Geometry check sheet. Reference: the model listing, model coordinates, mm. A direction names the side the tool comes from. Coordinates: 2 decimals unless noted, no trailing zeros. Write each loop counter-clockwise with the first axis right and the second up, starting at its lowest first coordinate (ties: lowest second). Pieces come first, ordered by that corner, then holes. Notation, with made-up numbers: M 50,5 L 104,5 A25 ccw 104,39 Z; hole C 45,5 d1. An arc over 180 degrees is marked long. Write each question's results on one line, items separated by ' | '.
Autodesk Inventor part; units mm, degrees
ref_plane "YZ Plane" through (0, 0, 0) normal (1, 0, 0) x (0, 1, 0)
ref_plane "XZ Plane" through (0, 0, 0) normal (0, 1, 0) x (-1, 0, 0)
ref_plane "XY Plane" through (0, 0, 0) normal (0, 0, 1) x (1, 0, 0)
sketch "Sketch1" plane through (0, 0, 0) normal (0, 1, 0) x (-1, 0, 0)
  line L0 (0, 0) -> (180, 0)
  line L1 (180, 0) -> (180, -60)
  line L2 (180, -60) -> (0, -60)
  line L3 (0, -60) -> (0, 0)
  dimension "d0" = 180
  dimension "d34" = 60
extrude "Plate1" add sketch "Sketch1" along normal blind 3
sketch "Sketch2" plane through (0, 3, 0) normal (0, 1, 0) x (1, 0, 0)
  line L0 (0, 60) -> (0, 0)
  line L1 (-180, 0) -> (-180, 60)
  line L2 (-133, 18.2) -> (-47, 18.2) construction
  line L3 (-180, 60) -> (0, 60) construction
  circle A0 centre (-103, 147.6372) radius 2
  circle A1 centre (-47, 147.6372) radius 2
  line L4 (-40, 142.6372) -> (-110, 142.6372)
  line L5 (-110, 142.6372) -> (-110, 152.6372)
  line L6 (-110, 152.6372) -> (-40, 152.6372)
  line L7 (-40, 152.6372) -> (-40, 142.6372)
  circle A2 centre (-103, 162.6372) radius 2
  circle A3 centre (-47, 162.6372) radius 2
  line L8 (-40, 157.6372) -> (-110, 157.6372)
  line L9 (-110, 157.6372) -> (-110, 167.6372)
  line L10 (-110, 167.6372) -> (-40, 167.6372)
  line L11 (-40, 167.6372) -> (-40, 157.6372)
  circle A4 centre (-103, 177.6372) radius 2
  circle A5 centre (-47, 177.6372) radius 2
  line L12 (-110, 182.6372) -> (-40, 182.6372)
  line L13 (-40, 182.6372) -> (-40, 172.6372)
  line L14 (-40, 172.6372) -> (-110, 172.6372)
  line L15 (-110, 172.6372) -> (-110, 182.6372)
  circle A6 centre (-103, 192.6372) radius 2
  circle A7 centre (-47, 192.6372) radius 2
  line L16 (-40, 187.6372) -> (-110, 187.6372)
  line L17 (-110, 187.6372) -> (-110, 197.6372)
  line L18 (-110, 197.6372) -> (-40, 197.6372)
  line L19 (-40, 197.6372) -> (-40, 187.6372)
  point P0 (-47, 10)
  point P1 (-133, 10)
  point P2 (-90, 18.2)
  point P3 (-90, 60)
  dimension "d4" = 8.2
  dimension "d31" = 86
  dimension "d56" = 10
hole "Hole1" at (-47, 3, -18.2) at (-47, 3, -10) at (-133, 3, -18.2) at (-133, 3, -10) direction (0, -1, 0) diameter 4 end through all
ref_plane "Work Plane1" through (-90, 0, 0) normal (1, 0, 0) x (0, 0, -1)
sketch "Sketch8" plane through (0, 0, 0) normal (0, -1, 0) x (1, 0, 0)
  line L0 (-180, 0) -> (-180, -60)
  line L1 (0, 0) -> (-180, 0)
  line L2 (-180, -60) -> (0, -60)
  line L3 (0, -60) -> (0, 0)
  line L4 (-175, -55) -> (-175, -5) construction
  line L5 (-175, -5) -> (-5, -5) construction
  line L6 (-5, -5) -> (-5, -55) construction
  line L7 (-5, -55) -> (-175, -55) construction
  dimension "d57" = 5
hole "Hole3" at (-175, 0, -5) at (-175, 0, -55) at (-5, 0, -55) at (-5, 0, -5) direction (0, 1, 0) diameter 4 end through all
sketch "Sketch9" plane through (0, 0, -60) normal (0, 0, -1) x (-1, 0, 0)
  line L0 (0, 0) -> (180, 0)
  line L1 (163, 0) -> (160, 0)
  line L2 (160, 0) -> (160, -120)
  line L3 (160, -120) -> (163, -120)
  line L4 (163, -120) -> (163, 0)
  line L5 (17, 0) -> (20, 0)
  line L6 (20, 0) -> (20, -120)
  line L7 (20, -120) -> (17, -120)
  line L8 (17, -120) -> (17, 0)
  line L9 (160, -120) -> (20, -120) construction
  point P0 (90, -120)
  point P1 (90, 0)
  dimension "d65" = 3
  dimension "d66" = 140
  dimension "d67" = 120
extrude "Extrusion3" add sketch "Sketch9" against normal blind 260
sketch "Sketch10" plane through (-17, -120, -60) normal (1, 0, 0) x (0, 0, -1)
  line L0 (-15, 15) -> (-15, 105)
  line L1 (-15, 105) -> (-101.675, 105)
  line L2 (-101.675, 105) -> (-15, 15)
  line L3 (-35.825, 15) -> (-122.5, 105)
  line L4 (-122.5, 105) -> (-122.5, 15)
  line L5 (-122.5, 15) -> (-35.825, 15)
  line L6 (-137.5, 15) -> (-137.5, 105)
  line L7 (-137.5, 105) -> (-224.175, 15)
  line L8 (-224.175, 15) -> (-137.5, 15)
  line L9 (-245, 15) -> (-158.325, 105)
  line L10 (-158.325, 105) -> (-245, 105)
  line L11 (-245, 105) -> (-245, 15)
  line L12 (-260, 0) -> (-260, 120)
  line L13 (-60, 120) -> (-260, 120)
  line L14 (0, 120) -> (0, 0)
  line L15 (0, 0) -> (-260, 0)
  point P0 (-8, 8)
  point P1 (-252, 8)
  point P2 (-252, 112)
  point P3 (-130, 8)
  point P4 (-130, 0)
  dimension "d70" = 15
  dimension "d71" = 15
  dimension "d72" = 15
  dimension "d73" = 15
  dimension "d74" = 15
  dimension "d75" = 15
  dimension "d77" = 15
  dimension "d80" = 8
  dimension "d81" = 8
  dimension "d82" = 8
  dimension "d83" = 8
extrude "Extrusion4" cut sketch "Sketch10" against normal through all
hole "Hole4" at (-17, -112, -52) at (-17, -112, 192) at (-17, -8, 192) at (-17, -112, 70) direction (-1, 0, 0) diameter 4 end through all
equation "\"d10\" = Thickness"
equation "\"d63\" = Thickness"
equation "\"BendRadius\" = Thickness"
equation "\"BendReliefWidth\" = Thickness"
equation "\"BendReliefDepth\" = 0.5 * Thickness"
equation "\"CornerReliefSize\" = 4 * Thickness"
equation "\"MinimumRemnant\" = 2 * Thickness"
equation "\"TransitionRadius\" = BendRadius"
equation "\"JacobiRadiusSize\" = BendRadius"
equation "\"GapSize\" = Thickness"
equation "\"d2\" = BendRadius"
properties part number "BASE"
Q1. Mould release check, pull along Z, two halves, no side actions. Record for faces 1 (the flat face through (-18.479, -59.37, -1.056)), 2 (the flat face through (-160, -59, 68)), 3 (the flat face through (-18.48, -60.63, 142.27)), 4 (the flat face through (-57.1, 0.4, -60)): pulls with the +Z half, pulls with the -Z half, needs draft (parallel to the pull), parting line crosses it, or undercut.
Geometry check:
face 1: undercut | face 2: needs draft | face 3: undercut | face 4: pulls with the -Z half
Q2. Sectioned sample at A-A on z = -32.5. Record the cut outline in (x, y), and give its area (3 significant figures).
Geometry check:
outline: M -180,0 L -163,0 L -163,-15 L -160,-15 L -160,0 L -20,0 L -20,-15 L -17,-15 L -17,0 L 0,0 L 0,3 L -180,3 Z; M -163,-120 L -160,-120 L -160,-92.02 L -163,-92.02 Z; M -20,-120 L -17,-120 L -17,-92.02 L -20,-92.02 Z | area: 798 mm2
Q3. Sectioned sample at C-C on y = -58. Give the number of separate pieces and of enclosed holes in the cut face, and give its area (3 significant figures).
Geometry check:
separate pieces: 10 | enclosed holes: 0 | area: 520 mm2
Q4. Access from +Z, -Z, +X, -X, +Y, -Y to the whole of each face (thin tool, end or side, straight path). Record for faces 5 (the flat face through (-20, -59, 68)), 6 (the flat face through (-163, -61, 68)), 7 (the flat face through (-161.48, -60.63, 142.27)).
Geometry check:
face 5: +Z, -Z, -Y | face 6: +Z, -Z, -X, -Y | face 7: +X, -X
Q5. Sectioned sample at D-D on x = -122.5. Record the cut outline in (y, z).
Geometry check:
outline: M 0,-60 L 3,-60 L 3,0 L 0,0 Z
Q6. Scan lines: probe 1 along X at (y, z) = (1.4, -55); probe 2 along Z at (x, y) = (-175, 1); probe 3 along X at (y, z) = (1, -18). Record each from-to range of solid material in increasing order.
Geometry check:
probe 1: x = -180 to -177, -173 to -7, -3 to 0 | probe 2: z = -60 to -57, -53 to -7, -3 to 0 | probe 3: x = -180 to -134.99, -131.01 to -48.99, -45.01 to 0
Q7. Sectioned sample at B-B on z = 8. Record the cut outline in (x, y), and give its area (3 significant figures).
Geometry check:
outline: M -163,-120 L -160,-120 L -160,-105 L -163,-105 Z; M -163,-71.59 L -160,-71.59 L -160,-49.97 L -163,-49.97 Z; M -163,-15 L -160,-15 L -160,0 L -163,0 Z; M -20,-120 L -17,-120 L -17,-105 L -20,-105 Z; M -20,-71.59 L -17,-71.59 L -17,-49.97 L -20,-49.97 Z; M -20,-15 L -17,-15 L -17,0 L -20,0 Z | area: 310 mm2
Q8. Depth check by flat-ended pin: P1, Ø6, axis at y = -53, z = 119.5, coming from the -X side; P2, Ø5, axis at x = -12, z = -27.5, coming from the -Y side; P3, Ø2.5, axis at x = -175, z = -5, coming from the +Y side; P4, Ø2.5, axis at x = -161.5, z = 116.5, coming from the +Y side. Enter the tip coordinate at first touch or a pass-through.
Geometry check:
P1: stops at x = -163 | P2: stops at y = 0 | P3: passes through | P4: stops at y = 0
